Build history of the part. All positions in model axes, mm. Face numbers are marked on the shaded views. Round coordinates to 2 decimals unless told otherwise and drop trailing zeros. Order: outer loops, then holes, each group sorted by start corner. A loop starts at its lowest first (then second) coordinate and runs counter-clockwise, first axis right, second up. Notation, with made-up numbers: M 79.25,-30.75 L 92.25,-30.75 A10 ccw 92.25,-11.75 Z; hole C 57,84 d11. An arc over 180 degrees is marked long. Use CSV: the item, a comma, the result in double quotes.
from build123d import *

# Parameters (mm, degrees)
BOSS_EXTRUDE1_DEPTH = 1.2
SKETCH2_R           = 3.5
BOSS_EXTRUDE2_DEPTH = 2.1
SKETCH3_R           = 2.5
CUT_EXTRUDE1_DEPTH  = 1
SKETCH4_R           = 1
CUT_EXTRUDE2_DEPTH  = 21.78090329
SKETCH6_R           = 2.45
CUT_EXTRUDE3_DEPTH  = 2.1
SKETCH7_R           = 0.5
CUT_EXTRUDE4_DEPTH  = 21.915208379
SKETCH8_R           = 0.5
CUT_EXTRUDE5_DEPTH  = 21.915208379


with BuildPart() as part:
    # Sketch1 → Boss-Extrude1 (new body)
    with BuildSketch(Plane.XY):
        with BuildLine():
            Line((-2, -6.75), (-2, -3))
            Line((-2, -3), (-14, -1.9))
            ThreePointArc((-14, -1.9), (-15.733799273, 0), (-14, 1.9))
            Line((-14, 1.9), (-2, 3))
            Line((-2, 3), (-2, 6.75))
            ThreePointArc((-2, 6.75), (0, 8.75), (2, 6.75))
            Line((2, 6.75), (2, 3.5))
            Line((2, 3.5), (17, 1.9))
            ThreePointArc((17, 1.9), (18.708111651, 0), (17, -1.9))
            Line((17, -1.9), (2, -3.5))
            Line((2, -3.5), (2, -6.75))
            ThreePointArc((2, -6.75), (0, -8.75), (-2, -6.75))
        make_face()
    extrude(amount=BOSS_EXTRUDE1_DEPTH)

    # Sketch2 → Boss-Extrude2 (add)
    with BuildSketch(Plane(origin=(0, 0, 0), x_dir=(-1, 0, 0), z_dir=(0, 0, -1))):
        Circle(SKETCH2_R)
    extrude(amount=BOSS_EXTRUDE2_DEPTH)

    # Sketch3 → Cut-Extrude1 (cut)
    with BuildSketch(Plane.XY.offset(1.2)):
        Circle(SKETCH3_R)
    extrude(amount=-CUT_EXTRUDE1_DEPTH, mode=Mode.SUBTRACT)

    # Sketch4 → Cut-Extrude2 (cut, through all)
    with BuildSketch(Plane.XY.offset(0.2)):
        Circle(SKETCH4_R)
    extrude(amount=-CUT_EXTRUDE2_DEPTH, mode=Mode.SUBTRACT)

    # Sketch6 → Cut-Extrude3 (cut)
    with BuildSketch(Plane(origin=(0, 0, -2.1), x_dir=(-1, 0, 0), z_dir=(0, 0, -1))):
        Circle(SKETCH6_R)
    extrude(amount=-CUT_EXTRUDE3_DEPTH, mode=Mode.SUBTRACT)

    # Sketch7 → Cut-Extrude4 (cut, through all)
    with BuildSketch(Plane.XY.offset(1.2)):
        with Locations((0, -4.5)):
            Circle(SKETCH7_R)
        with Locations((0, -6.5)):
            Circle(SKETCH7_R)
        with Locations((0, 4.5)):
            Circle(SKETCH7_R)
        with Locations((0, 6.5)):
            Circle(SKETCH7_R)
    extrude(amount=-CUT_EXTRUDE4_DEPTH, mode=Mode.SUBTRACT)

    # Sketch8 → Cut-Extrude5 (cut, through all)
    with BuildSketch(Plane.XY.offset(1.2)):
        with Locations((-4.5, 0)):
            Circle(SKETCH8_R)
        with Locations((-6.5, 0)):
            Circle(SKETCH8_R)
        with Locations((-8.5, 0)):
            Circle(SKETCH8_R)
        with Locations((-10.5, 0)):
            Circle(SKETCH8_R)
        with Locations((-12.5, 0)):
            Circle(SKETCH8_R)
        with Locations((-14.5, 0)):
            Circle(SKETCH8_R)
        with Locations(Location((4.5, 0, 0), (0, 0, 180))):
            Circle(SKETCH8_R)
        with Locations(Location((6.5, 0, 0), (0, 0, 180))):
            Circle(SKETCH8_R)
        with Locations(Location((8.5, 0, 0), (0, 0, 180))):
            Circle(SKETCH8_R)
        with Locations(Location((10.5, 0, 0), (0, 0, 180))):
            Circle(SKETCH8_R)
        with Locations(Location((12.5, 0, 0), (0, 0, 180))):
            Circle(SKETCH8_R)
        with Locations(Location((14.5, 0, 0), (0, 0, 180))):
            Circle(SKETCH8_R)
        with Locations((16.5, 0)):
            Circle(SKETCH8_R)
    extrude(amount=-CUT_EXTRUDE5_DEPTH, mode=Mode.SUBTRACT)


solid = part.part
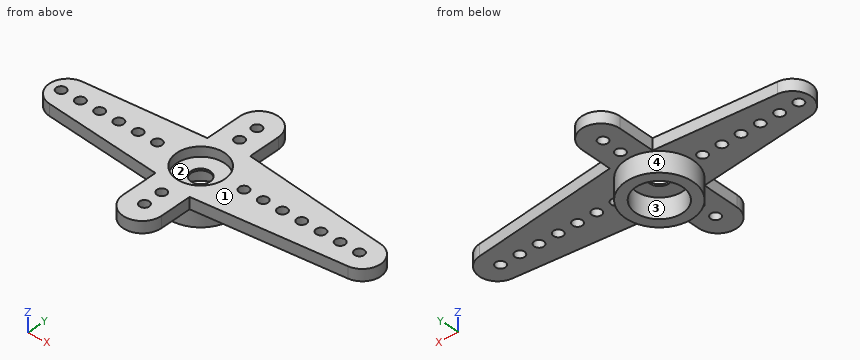
(1) Wall check: line 1 (Y direction, x = 0, z = 0.9); line 2 (Z direction, x = 17, y = -1.75); line 3 (Y direction, x = 0.5, z = -0.05). Give the ranges that are in metal, low to high. Write a range as from..to.
Answer block:
line 1,"y = -8.75..-7, -6..-5, -4..-2.5, 2.5..4, 5..6, 7..8.75"
line 2,"z = 0..1.2"
line 3,"y = -3.46..-2.4, 2.4..3.46"
(2) Cut at C-C, the plane x = 0. Count the separate pieces of the cut face and the enclosed holes in it, and give its area (3 significant figures).
Answer block:
separate pieces,"6"
enclosed holes,"0"
area,"15.2 mm²"
(3) Cut at D-D, the plane z = -1.2. Give the cut face in (x, y).
Answer block:
outline,"C 0,0 d7; hole C 0,0 d4.9"
(4) Two-plate mould, pull along X, no slides. Class the marked faces 1, 2, 3 and 4: released by +X, released by -X, zero draft, split by the parting line, or undercut.
Answer block:
face 1,"zero draft"
face 2,"undercut"
face 3,"undercut"
face 4,"split by the parting line"
(5) Drop flat-ended pins along their axis: pin 1 (1.5 mm diameter, centred on x = 15, y = 0, fed in from -Z); pin 2 (2.5 mm diameter, centred on x = 0, y = 0, fed in from +Z); pin 3 (1.5 mm diameter, centred on x = 5.5, z = -0.5, fed in from +Y). Give the stop position or say it passes through.
Answer block:
pin 1,"stops at z = 0"
pin 2,"stops at z = 0.2"
pin 3,"stops at y = 3.19"
(6) Cut at A-A, the plane y = 4.5. Give the cut face in (x, z), and give its area (3 significant figures).
Answer block:
outline,"M -2,0 L -0.5,0 L -0.5,1.2 L -2,1.2 Z; M 0.5,0 L 2,0 L 2,1.2 L 0.5,1.2 Z"
area,"3.60 mm²"
(7) Cut at B-B, the plane x = -6.5. Give the cut face in (y, z).
Answer block:
outline,"M -2.59,0 L -0.5,0 L -0.5,1.2 L -2.59,1.2 Z; M 0.5,0 L 2.59,0 L 2.59,1.2 L 0.5,1.2 Z"
